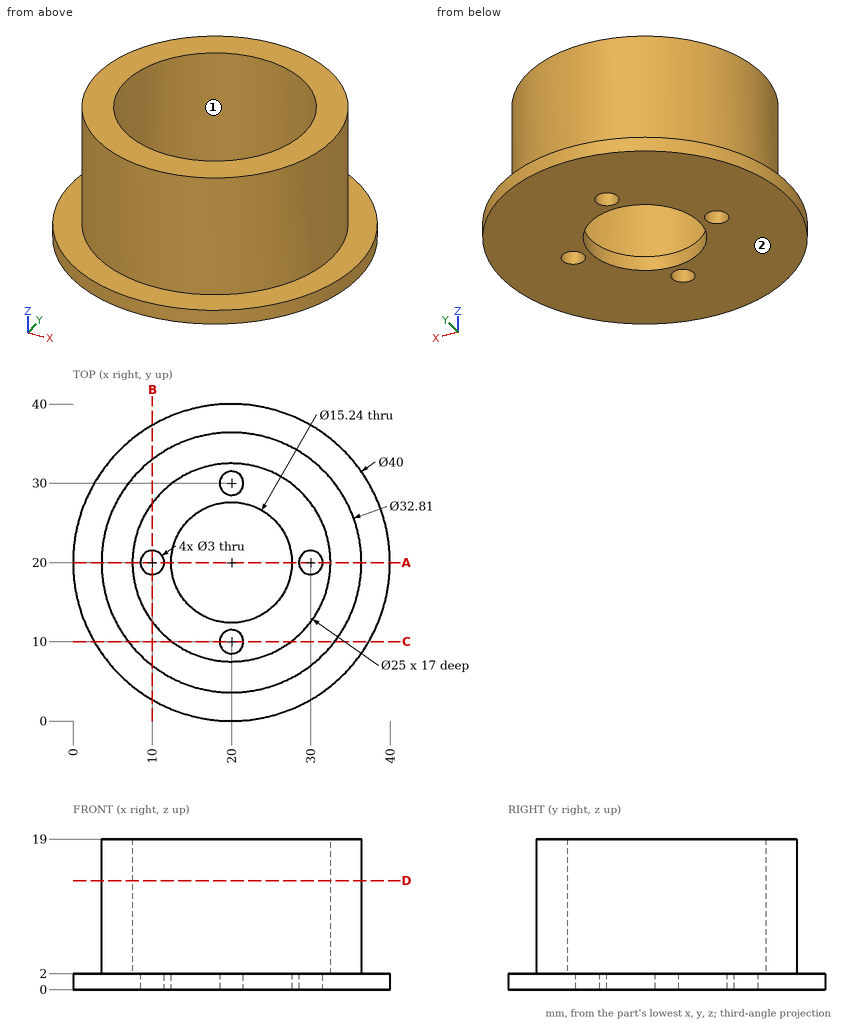
Geometry check sheet. Reference: drawing and pictorial views, mm from the part's lowest x, y, z. A direction names the side the tool comes from. Give positions to 0.01 mm unless a question says otherwise; leave off trailing zeros. Order: outer loops, then holes, each group sorted by start corner. A loop starts at its lowest first (then second) coordinate and runs counter-clockwise, first axis right, second up. Notation, with made-up numbers: (77.5, -30) -> (115.5, -30) arc R29 ccw to (115.5, 0) -> close; hole circle Ø2 at (37, 7). An arc over 180 degrees is marked (long way). Use CSV: the item, a comma, the result in double quotes. Start each with the question number.
1) Material ranges on line 1 (Y direction, x = 20, z = 1.4); line 2 (Y direction, x = 20, z = 7.25) (3 decimals); line 3 (Z direction, x = 3, y = 26), recorded low to high. Write a range as from..to.
2) Sectioned sample at D-D, the plane z = 13.75. Record the boundary of the cut face in (x, y) (3 decimals).
3) Set-up check for the marked faces 1 and 2: record each of +Z, -Z, +X, -X, +Y, -Y from which the full face is reachable in a straight line by a thin tool's end or side.
4) Go/stop test with flat-tipped pins: P1, Ø1, axis at y = 7, z = 9.5, coming from the +X side; P2, Ø12, axis at x = 14, y = 21.5, coming from the +Z side; P3, Ø3, axis at y = 33, z = 9.5, coming from the -X side; P4, Ø1.8, axis at x = 10, y = 20, coming from the +Z side. Record where each tip stops, or that it passes through.
5) Sectioned sample at B-B, the plane x = 10. Record the boundary of the cut face in (y, z).
6) Sectioned sample at A-A, the plane y = 20. Record the boundary of the cut face in (x, z) (3 decimals), plus the area to 3 significant figures.
Recorded:
1,line 1,"0..8.5, 11.5..12.38, 27.62..28.5, 31.5..40"
1,line 2,"3.595..7.5, 32.5..36.405"
1,line 3,"0..2"
2,outline,"circle Ø32.81 at (20, 20); hole circle Ø25 at (20, 20)"
3,face 1,"+Z"
3,face 2,"-Z, +X, -X, +Y, -Y"
4,P1,"x = 30.62"
4,P2,"z = 2"
4,P3,"x = 8.3"
4,P4,"through"
5,outline,"(2.68, 0) -> (18.5, 0) -> (18.5, 2) -> (12.5, 2) -> (12.5, 19) -> (7, 19) -> (7, 2) -> (2.68, 2) -> close; (21.5, 0) -> (37.32, 0) -> (37.32, 2) -> (33, 2) -> (33, 19) -> (27.5, 19) -> (27.5, 2) -> (21.5, 2) -> close"
6,outline,"(0, 0) -> (8.5, 0) -> (8.5, 2) -> (7.5, 2) -> (7.5, 19) -> (3.595, 19) -> (3.595, 2) -> (0, 2) -> close; (11.5, 0) -> (12.38, 0) -> (12.38, 2) -> (11.5, 2) -> close; (27.62, 0) -> (28.5, 0) -> (28.5, 2) -> (27.62, 2) -> close; (31.5, 0) -> (40, 0) -> (40, 2) -> (36.405, 2) -> (36.405, 19) -> (32.5, 19) -> (32.5, 2) -> (31.5, 2) -> close"
6,area,"170 mm2"
